Autodesk Inventor part; units mm, degrees
ref_plane "YZ Plane" through (0, 0, 0) normal (1, 0, 0) x (0, 1, 0)
ref_plane "XZ Plane" through (0, 0, 0) normal (0, 1, 0) x (-1, 0, 0)
ref_plane "XY Plane" through (0, 0, 0) normal (0, 0, 1) x (1, 0, 0)
sketch "Szkic1" plane through (0, 0, 0) normal (0, 1, 0) x (-1, 0, 0)
  circle A0 centre (0, 0) radius 36.5
  circle A1 centre (0, 0) radius 32.5
  circle A2 centre (0, 0) radius 5
  circle A3 centre (0, 0) radius 1.65
  line L0 (1.15, 1.1832) -> (1.15, -1.1832)
  line L1 (-4.9328, 0.8172) -> (-25.2334, 20.4824)
  line L2 (-11.5454, 30.3802) -> (0.8172, 4.9328)
  line L3 (-4.9328, 0.8172) -> (-30.3802, -11.5454)
  line L4 (4.9328, -0.8172) -> (25.2334, -20.4824)
  line L5 (0.8172, 4.9328) -> (20.4824, 25.2334)
  line L6 (4.9328, -0.8172) -> (30.3802, 11.5454)
  line L7 (-0.8172, -4.9328) -> (-20.4824, -25.2334)
  line L8 (-0.8172, -4.9328) -> (11.5454, -30.3802)
  dimension "d1" = 65
  dimension "d0" = 73
  dimension "d2" = 10
  dimension "d3" = 3.3
  dimension "d4" = 2.8
  dimension "d6" = 20
  dimension "d7" = 20
  dimension "d14" = 20
  dimension "d15" = 20
  dimension "d16" = 5.75
  dimension "d17" = 5.75
  dimension "d18" = 5.75
  dimension "d19" = 5.75
  dimension "d20" = 70
  dimension "d21" = 70
  dimension "d22" = 70
extrude "Wyciągnięcie proste1" add sketch "Szkic1" along normal blind 9 contours A0 | L6 A2 L5 A1 | A1 L8 A2 L4 | A2 | L2 A2 L1 A1 | L7 A1 L3 A2 | A3 L0 picked at (1.3167, 0)
properties part number "kolko1"
For this review, take the finished solid that the model builds, in its own axes (mm). A direction names the side the tool comes from. Give positions to 0.01 mm unless a question says otherwise; leave off trailing zeros. Write each loop counter-clockwise with the first axis right and the second up, starting at its lowest first coordinate (ties: lowest second). Pieces come first, ordered by that corner, then holes.
Item 1: Take a section at C-C (z = 19.5). Give the boundary of the cut face in (x, y).
Item 2: Take a section at A-A (z = 27). Give the boundary of the cut face in (x, y), and give its area (3 significant figures).
Item 3: Wall thickness on probe 1 along Z at (x, y) = (0.5, 7.75); probe 2 along Z at (x, y) = (0, 4.75); probe 3 along X at (y, z) = (1, 11): over which ranges is each line inside the solid? List them lowest first.
Item 4: The part is to be moulded in two halves that separate along X. For faces 3 (the face through (-8, 9, 1)), 4 (the face through (-10.51, 4.44, 14.94)), 5 (the face through (7.912, 4.437, 35.632)), say which applies: +X half, -X half, draft (parallel to the pull), parting line (faces both ways), or undercut.
Item 5: Machinability: for faces 1 (the face through (-5.28, 4.44, -17.48)), 2 (the face through (-8, 0, 1)), which of the approach directions +Z, -Z, +X, -X, +Y, -Y give a long, thin tool a straight path to every point of the face, cutting with its end or side? Answer none if there is none.
Item 6: Take a section at D-D (y = 3.5). Give the boundary of the cut face in (x, z).
Item 7: Take a section at B-B (x = 22). Give the boundary of the cut face in (y, z).
Item 8: Insertion check: P1, Ø3, axis at x = 23.5, y = 6.5, coming from the +Z side; P2, Ø1.2, axis at y = 6, z = -0.5, coming from the +X side; P3, Ø3, axis at x = 6, y = 4.5, coming from the -Z side; P4, Ø5, axis at x = 25.5, y = 3, coming from the -Z side. Each pin has a flat end and moves straight along its axis. Give the tip position at first contact, or say it passes through.
Established:
1. outline: (-30.85, 0) - (-14.93, 0) - (-14.93, 9) - (-30.85, 9) - close; (6.26, 0) - (24.22, 0) - (24.22, 9) - (6.26, 9) - close; (26, 0) - (30.85, 0) - (30.85, 9) - (26, 9) - close
2. outline: (-24.56, 0) - (-18.09, 0) - (-18.09, 9) - (-24.56, 9) - close; (9.9, 0) - (24.56, 0) - (24.56, 9) - (9.9, 9) - close
2. area: 190 mm2
3. probe 1: z = -36.5 to -32.5, -5.59 to -1.57, 1.57 to 7.64, 32.5 to 36.5
3. probe 2: z = -36.5 to -32.5, -6.61 to -1.65, 1.65 to 6.61, 32.5 to 36.5
3. probe 3: x = -34.8 to -30.58, -29.26 to -6.69, 2.13 to 15.44, 30.58 to 34.8
4. face 3: draft
4. face 4: undercut
4. face 5: parting line
5. face 1: +Y, -Y
5. face 2: +Z, -Z, +X, -X, -Y
6. outline: circle Ø73 at (0, 0); hole (-30.38, 11.55) arc R32.5 ccw to (-25.23, -20.48) - (-4.93, -0.82) - close; hole (-20.48, 25.23) - (-0.82, 4.93) - (11.55, 30.38) arc R32.5 ccw to start; hole (-11.55, -30.38) arc R32.5 ccw to (20.48, -25.23) - (0.82, -4.93) - close; hole (-1.15, -1.18) arc R1.65 ccw (long way) to (-1.15, 1.18) - close; hole (4.93, 0.82) - (30.38, -11.55) arc R32.5 ccw to (25.23, 20.48) - close
7. outline: (0, -29.12) - (9, -29.12) - (9, -7.47) - (0, -7.47) - close; (0, 17.35) - (9, 17.35) - (9, 29.12) - (0, 29.12) - close
8. P1: stops at z = 29.12
8. P2: stops at x = 36.5
8. P3: stops at z = -36.22
8. P4: stops at z = -28.34
